Source: CAD feature listing. Evaluate the final solid. Frame: model axes, mm. Round coordinates to 2 decimals unless told otherwise and drop trailing zeros. Write each loop counter-clockwise with the first axis right and the second up, starting at its lowest first coordinate (ties: lowest second). Pieces come first, ordered by that corner, then holes. Notation, with made-up numbers: (-28.5, 4) -> (23.5, 4) arc R13 ccw to (23.5, 27) -> close; hole circle Ø6 at (3.25, 34). An arc over 180 degrees is marked (long way). Return JSON: item names as keys, results as strings. Group by question number.
from build123d import *

# Parameters (mm, degrees)
ESBO_O1_W                = 20
ESBO_O1_H                = 40
ESBO_O1_W_2              = 16
ESBO_O1_H_2              = 36
RESSALTO_EXTRUS_O1_DEPTH = 340
ESBO_O2_R                = 1.75
CORTE_EXTRUS_O1_DEPTH    = 2
ESBO_O3_R                = 3
CORTE_EXTRUS_O2_DEPTH    = 2
ESBO_O4_R                = 4.25
CORTE_EXTRUS_O3_DEPTH    = 2


with BuildPart() as part:
    # Esboço1 → Ressalto-extrusão1 (new body)
    with BuildSketch(Plane.XY):
        with Locations((10, 20)):
            Rectangle(ESBO_O1_W, ESBO_O1_H)
        with Locations((10, 20)):
            Rectangle(ESBO_O1_W_2, ESBO_O1_H_2, mode=Mode.SUBTRACT)
    extrude(amount=RESSALTO_EXTRUS_O1_DEPTH)

    # Esboço2 → Corte-extrusão1 (cut)
    with BuildSketch(Plane.ZY):
        with Locations((10, 30)):
            Circle(ESBO_O2_R)
        with Locations((10, 15)):
            Circle(ESBO_O2_R)
        with Locations((70, 15)):
            Circle(ESBO_O2_R)
        with Locations((55, 15)):
            Circle(ESBO_O2_R)
        with Locations(Location((270, 15, 0), (0, 0, 180))):
            Circle(ESBO_O2_R)
        with Locations(Location((285, 15, 0), (0, 0, 180))):
            Circle(ESBO_O2_R)
        with Locations(Location((330, 15, 0), (0, 0, 180))):
            Circle(ESBO_O2_R)
        with Locations(Location((330, 30, 0), (0, 0, 180))):
            Circle(ESBO_O2_R)
    extrude(amount=-CORTE_EXTRUS_O1_DEPTH, mode=Mode.SUBTRACT)

    # Esboço3 → Corte-extrusão2 (cut)
    with BuildSketch(Plane(origin=(0, 40, 0), x_dir=(1, 0, 0), z_dir=(0, 1, 0))):
        with Locations(Location((10, -320, 0), (0, 0, 270))):
            Circle(ESBO_O3_R)
        with Locations(Location((10, -20, 0), (0, 0, 90))):
            Circle(ESBO_O3_R)
    extrude(amount=-CORTE_EXTRUS_O2_DEPTH, mode=Mode.SUBTRACT)

    # Esboço4 → Corte-extrusão3 (cut)
    with BuildSketch(Plane(origin=(20, 0, 0), x_dir=(0, 0, -1), z_dir=(1, 0, 0))):
        with Locations((-320, 20)):
            Circle(ESBO_O4_R)
        with Locations(Location((-20, 20, 0), (0, 0, 180))):
            Circle(ESBO_O4_R)
    extrude(amount=-CORTE_EXTRUS_O3_DEPTH, mode=Mode.SUBTRACT)


solid = part.part
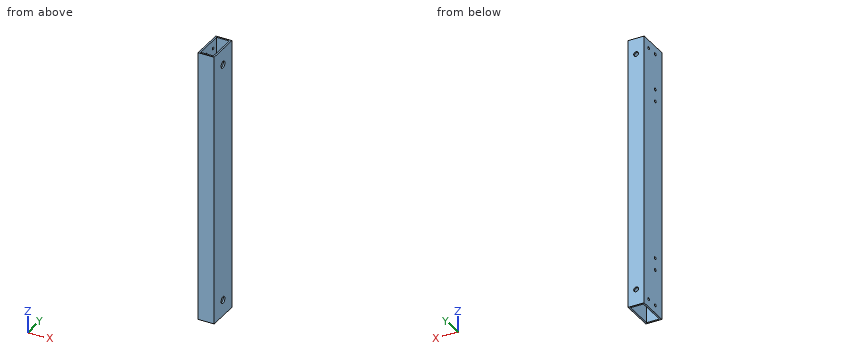
Item 1: Cut plane B-B on z = 89.5. Output: boundary loops of the cut face in (x, y).
Item 2: Cut plane A-A on x = 10. Output: boundary loops of the cut face in (y, z), and give its area (3 significant figures).
Item 3: Material intervals for probe 1 along Y at (x, z) = (0.6, 330); probe 2 along Y at (x, z) = (5.25, 44); probe 3 along X at (y, z) = (18.5, 178), sorted ascending.
Item 4: First-contact query: pin 1 Ø10 at (y, z) = (20, 320) entering from +X; pin 2 Ø3 at (y, z) = (15, 330) entering from -X. Flat tips, straight axial feed; report the tip coordinate or a pass-through.
Item 5: Cut plane D-D on y = 6. Output: boundary loops of the cut face in (x, z).
Item 6: Cut plane C-C on y = 20. Output: boundary loops of the cut face in (x, z).
Here are the results:
{
 "1": {"outline": "(0, 0) -> (20, 0) -> (20, 40) -> (0, 40) -> close; hole (2, 2) -> (18, 2) -> (18, 38) -> (2, 38) -> close"},
 "2": {"outline": "(0, 0) -> (2, 0) -> (2, 340) -> (0, 340) -> close; (38, 0) -> (40, 0) -> (40, 17) -> (38, 17) -> close; (38, 23) -> (40, 23) -> (40, 317) -> (38, 317) -> close; (38, 323) -> (40, 323) -> (40, 340) -> (38, 340) -> close", "area": "1,340 mm^2"},
 "3": {"probe 1": "y = 0 to 13.25, 16.75 to 28.25, 31.75 to 40", "probe 2": "y = 0 to 2, 38 to 40", "probe 3": "x = 0 to 2, 18 to 20"},
 "4": {"pin 1": "stops at x = 20", "pin 2": "stops at x = 18"},
 "5": {"outline": "(0, 0) -> (2, 0) -> (2, 340) -> (0, 340) -> close; (18, 0) -> (20, 0) -> (20, 340) -> (18, 340) -> close"},
 "6": {"outline": "(0, 0) -> (2, 0) -> (2, 340) -> (0, 340) -> close; (18, 0) -> (20, 0) -> (20, 15.75) -> (18, 15.75) -> close; (18, 24.25) -> (20, 24.25) -> (20, 315.75) -> (18, 315.75) -> close; (18, 324.25) -> (20, 324.25) -> (20, 340) -> (18, 340) -> close"}
}
